Could you check a few things on this model? Use its own coordinates, in mm. A direction names the side the tool comes from. Round coordinates to 2 decimals unless told otherwise and drop trailing zeros. Loops run counter-clockwise (first coordinate to the right, second up) from the corner with the lowest first, then second, coordinate; pieces in that order, holes last. Notation, with made-up numbers: (-27.75, -3.5) -> (16.25, -3.5) arc R15 cw to (16.25, 16.5) -> close; hole circle Ø2 at (75.25, 80). An arc over 180 degrees is marked (long way). Write each question's results on one line, items separated by ' | '.
from build123d import *

# Parameters (mm, degrees)
SKETCH1_R           = 16.5
BOSS_EXTRUDE1_DEPTH = 1
SKETCH2_R           = 13.5
BOSS_EXTRUDE2_DEPTH = 3
SKETCH3_R           = 12
CUT_EXTRUDE1_DEPTH  = 3
SKETCH5_R           = 0.75
CUT_EXTRUDE3_DEPTH  = 17


with BuildPart() as part:
    # Sketch1 → Boss-Extrude1 (new body)
    with BuildSketch(Plane(origin=(0, 0, 0), x_dir=(1, 0, 0), z_dir=(0, 1, 0))):
        Circle(SKETCH1_R)
    extrude(amount=BOSS_EXTRUDE1_DEPTH)

    # Sketch2 → Boss-Extrude2 (add)
    with BuildSketch(Plane(origin=(0, 0, 0), x_dir=(1, 0, 0), z_dir=(0, 1, 0))):
        Circle(SKETCH2_R)
    extrude(amount=BOSS_EXTRUDE2_DEPTH)

    # Sketch3 → Cut-Extrude1 (cut)
    with BuildSketch(Plane(origin=(0, 0, 0), x_dir=(1, 0, 0), z_dir=(0, 1, 0))):
        Circle(SKETCH3_R)
    extrude(amount=CUT_EXTRUDE1_DEPTH, mode=Mode.SUBTRACT)

    # Sketch5 → Cut-Extrude3 (cut)
    with BuildSketch(Plane(origin=(0, 0, 0), x_dir=(0, 0, -1), z_dir=(1, 0, 0))):
        with Locations((0, 1.36)):
            Circle(SKETCH5_R)
    extrude(amount=CUT_EXTRUDE3_DEPTH, mode=Mode.SUBTRACT)


solid = part.part
1) I'm going to push flat-ended pins straight in: pin 1 (1.5 mm diameter, centred on y = 1.5, z = -7, fed in from -X); pin 2 (4 mm diameter, centred on x = -12.5, z = -9.5, fed in from +Y); pin 3 (1.5 mm diameter, centred on y = 2, z = -8, fed in from -X). Where does each tip first touch, or does it pass through?
Model answer:
pin 1: stops at x = -15.19 | pin 2: stops at y = 1 | pin 3: stops at x = -11.39
2) If we mould it in two halves opening along Y, with no side actions, what happens to faces 3 (the flat face through (1.15, 0, 12.15)), 4 (the cylindrical face through (13.704, 0.628, 0.163)), 5 (the flat face through (-12, 3, 2))? For each: released by +Y, released by -Y, zero draft, split by the parting line, or undercut.
Model answer:
face 3: released by -Y | face 4: undercut | face 5: released by +Y
3) I want a section at B-B, the plane x = 0. Write out the boundary of the cut face in (y, z), plus the area to 3 significant figures.
Model answer:
outline: (0, -16.5) -> (1, -16.5) -> (1, -13.5) -> (3, -13.5) -> (3, -12) -> (0, -12) -> close; (0, 12) -> (3, 12) -> (3, 13.5) -> (1, 13.5) -> (1, 16.5) -> (0, 16.5) -> close | area: 15.0 mm2
4) I want a section at A-A, the plane z = 0. Write out the boundary of the cut face in (x, y).
Model answer:
outline: (-16.5, 0) -> (-12, 0) -> (-12, 3) -> (-13.5, 3) -> (-13.5, 1) -> (-16.5, 1) -> close; (12, 0) -> (16.5, 0) -> (16.5, 0.61) -> (12, 0.61) -> close; (12, 2.11) -> (13.5, 2.11) -> (13.5, 3) -> (12, 3) -> close
5) I need wall thicknesses on line 1 (Z direction, x = 0, y = 1.9); line 2 (Y direction, x = 13, z = 0); line 3 (Z direction, x = 0, y = 0.6). Which ranges of each line are inside material? Lowest first, please.
Model answer:
line 1: z = -13.5 to -12, 12 to 13.5 | line 2: y = 0 to 0.61, 2.11 to 3 | line 3: z = -16.5 to -12, 12 to 16.5
6) For faces 1 (the cylindrical face through (-11.99, 1.48, -0.53)), 2 (the flat face through (0, 1, -14)), which set-ups out of +Z, -Z, +X, -X, +Y, -Y let a thin tool reach every point of the face, with its end or its side?
Model answer:
face 1: +Y, -Y | face 2: +Y
7) I want a section at D-D, the plane x = 13. Write out the boundary of the cut face in (y, z), plus the area to 3 significant figures.
Model answer:
outline: (0, -10.16) -> (1, -10.16) -> (1, -3.64) -> (3, -3.64) -> (3, 3.64) -> (1, 3.64) -> (1, 10.16) -> (0, 10.16) -> close; hole circle Ø1.5 at (1.36, 0) | area: 33.1 mm2
8) I want a section at C-C, the plane z = 3.5. Write out the boundary of the cut face in (x, y).
Model answer:
outline: (-16.12, 0) -> (-11.48, 0) -> (-11.48, 3) -> (-13.04, 3) -> (-13.04, 1) -> (-16.12, 1) -> close; (11.48, 0) -> (16.12, 0) -> (16.12, 1) -> (13.04, 1) -> (13.04, 3) -> (11.48, 3) -> close
